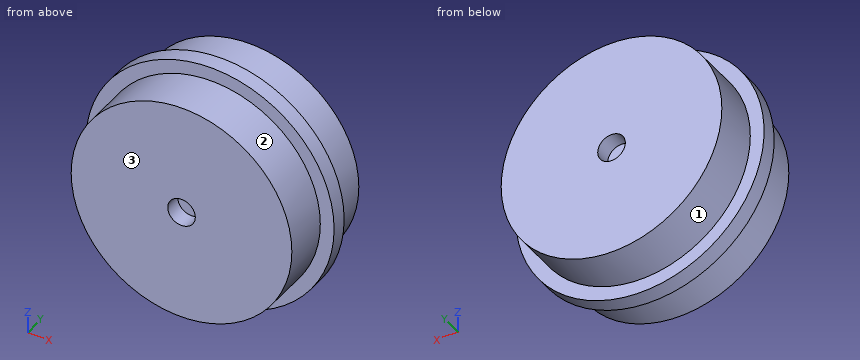
```python
from build123d import *

# Parameters (mm, degrees)
F0_R     = 20
F0_R_2   = 15
F1_DEPTH = 10
F3_R     = 22.5
F3_R_2   = 2.5
F4_DEPTH = 1.5
F7_R     = 15
F7_R_2   = 2.5
F8_DEPTH = 3


with BuildPart() as f1:
    # F0 (on Front) → F1 (new body)
    with BuildSketch(Plane.XZ):
        Circle(F0_R)
        Circle(F0_R_2, mode=Mode.SUBTRACT)
    extrude(amount=F1_DEPTH)

    # F2: F1 across plane


with BuildPart() as f1_1:
    add(f1.part)
    add(f1.part.mirror(Plane.XZ))

    # F3 (on Front) → F4 (join)
    with BuildSketch(Plane.XZ):
        Circle(F3_R)
        Circle(F3_R_2, mode=Mode.SUBTRACT)
    extrude(amount=F4_DEPTH)

    # F5: F1 across plane


with BuildPart() as f1_2:
    add(f1_1.part)
    add(f1_1.part.mirror(Plane.XZ))

    # F7 (on offset) → F8 (join)
    with BuildSketch(Plane.XZ.offset(10)):
        Circle(F7_R)
        Circle(F7_R_2, mode=Mode.SUBTRACT)
    extrude(amount=-F8_DEPTH)

    # F9: F1 across plane


with BuildPart() as f1_3:
    add(f1_2.part)
    add(f1_2.part.mirror(Plane.XZ))


solid = f1_3.part
```
Geometry check sheet. Reference: the model listing, model coordinates, mm. Face numbers are marked on the shaded views. A direction names the side the tool comes from. Give positions to 0.01 mm unless a question says otherwise; leave off trailing zeros. Order: outer loops, then holes, each group sorted by start corner. A loop starts at its lowest first (then second) coordinate and runs counter-clockwise, first axis right, second up. Notation, with made-up numbers: (23, -12.5) - (40, -12.5) arc R7 cw to (40, -0.5) - close; hole circle Ø11 at (5.5, 69.25). An arc over 180 degrees is marked (long way). Answer in a Markdown table with one row per item. Add a question column.
Q1. Tool access check on the marked faces 1, 2 and 3. Record the directions out of +Z, -Z, +X, -X, +Y, -Y that give a thin tool (end or side, any length) a straight path to the whole face; none if there is none.
Q2. Cross-section at C-C, the plane z = -8.5. Enter the section's corners in (x, y).
Q3. Cross-section at D-D, the plane x = -7.5. Enter the section's corners in (y, z), then the cut area to 3 significant figures.
Q4. Gauge pin test, flat ends, axial feed: pin 1 (12 mm diameter, centred on y = 0.5, z = -11.5, fed in from -X); pin 2 (1 mm diameter, centred on y = 1, z = -2.5, fed in from -X); pin 3 (1.5 mm diameter, centred on y = 6.5, z = -3.5, fed in from -X); pin 4 (4.5 mm diameter, centred on x = 0, z = 0, fed in from -Y). Record the tip position at first contact, or that the pin passes through.
Q5. Material ranges on probe 1 along Y at (x, z) = (-7, 9); probe 2 along Z at (x, y) = (0, 0.4); probe 3 along Z at (x, y) = (0, -9.25), recorded low to high. Write a range as from..to.
Check values:
| question | item | result |
|---|---|---|
| 1 | face 1 | +Y |
| 1 | face 2 | -Y |
| 1 | face 3 | +Z, -Z, +X, -X, -Y |
| 2 | outline | (-20.83, -1.5) - (-18.1, -1.5) - (-18.1, -10) - (18.1, -10) - (18.1, -1.5) - (20.83, -1.5) - (20.83, 1.5) - (18.1, 1.5) - (18.1, 10) - (-18.1, 10) - (-18.1, 1.5) - (-20.83, 1.5) - close; hole (-12.36, -7) - (12.36, -7) - (12.36, -1.5) - (-12.36, -1.5) - close; hole (-12.36, 1.5) - (12.36, 1.5) - (12.36, 7) - (-12.36, 7) - close |
| 3 | outline | (-10, -18.54) - (-1.5, -18.54) - (-1.5, -21.21) - (1.5, -21.21) - (1.5, -18.54) - (10, -18.54) - (10, 18.54) - (1.5, 18.54) - (1.5, 21.21) - (-1.5, 21.21) - (-1.5, 18.54) - (-10, 18.54) - close; hole (-7, -12.99) - (-1.5, -12.99) - (-1.5, 12.99) - (-7, 12.99) - close; hole (1.5, -12.99) - (7, -12.99) - (7, 12.99) - (1.5, 12.99) - close |
| 3 | area | 472 mm^2 |
| 4 | pin 1 | stops at x = -21.82 |
| 4 | pin 2 | stops at x = -22.41 |
| 4 | pin 3 | stops at x = -19.81 |
| 4 | pin 4 | passes through |
| 5 | probe 1 | y = -10..-7, -1.5..1.5, 7..10 |
| 5 | probe 2 | z = -22.5..-2.5, 2.5..22.5 |
| 5 | probe 3 | z = -20..-2.5, 2.5..20 |
